CAD build for the part. Positions are in the model's coordinates, mm. Give positions to 0.01 mm unless a question says otherwise; leave off trailing zeros. Loops run counter-clockwise (first coordinate to the right, second up) from the corner with the lowest first, then second, coordinate; pieces in that order, holes last.
Item 1: Mould opens along Z. For faces 1 (the cylindrical face through (7.543, -2.415, 14.114)), 2 (the cylindrical face through (12.499, -2.348, 6.005)), 3 (the flat face through (50.377, -0.825, 15.654)) say: released by +Z, released by -Z, zero draft, split by the parting line, or undercut.
Item 2: Saw through at D-D on z = 15.5. Give the cut face in (x, y) (1 decimal), plus the area to 3 significant figures.
Item 3: Saw through at B-B on y = -3.75. Give the cut face in (x, z).
Item 4: Drop flat-ended pins along their axis: P1, Ø3.5, axis at x = 7.94, z = 11.11, coming from the -Y side; P2, Ø4, axis at x = 49, z = 11.5, coming from the +Y side. Give the stop position or say it passes through.
Item 5: Saw through at C-C on x = 47.5. Give the cut face in (y, z).
Item 6: Probe probe 1 along Z at (x, y) = (7, -0.9); probe 2 along Z at (x, y) = (8, -1.35); probe 3 along Z at (x, y) = (15, -1.8). List the from-to ranges inside material, lowest first.
Item 7: Saw through at A-A on z = 9.5. Give the cut face in (x, y), plus the area to 3 significant figures.
from build123d import *

# Parameters (mm, degrees)
F1_DEPTH = 4.7625
F2_R     = 3.027234
F3_DEPTH = 25.4
F5_DEPTH = 25.4


with BuildPart() as f1:
    # F0 (on Front) → F1 (new body)
    with BuildSketch(Plane.XZ):
        with BuildLine():
            Line((60.325, 19.05), (7.914832, 19.05))
            ThreePointArc((7.914832, 19.05), (2.318201, 16.731799), (0, 11.135168))
            Line((0, 11.135168), (0, 0))
            Line((0, 0), (9.520886, 0.27992))
            Line((9.520886, 0.27992), (10.734157, 3.685592))
            ThreePointArc((10.734157, 3.685592), (12.533664, 6.029149), (15.364371, 6.876249))
            Line((15.364371, 6.876249), (60.325, 12.7))
            Line((60.325, 12.7), (60.325, 19.05))
        make_face()
    extrude(amount=F1_DEPTH)

    # F2 (on face) → F3 (cut)
    with BuildSketch(Plane.XZ.offset(4.7625)):
        with Locations((7.937468, 11.1125)):
            Circle(F2_R)
    extrude(amount=-F3_DEPTH, mode=Mode.SUBTRACT)

    # F4 (on face) → F5 (cut)
    with BuildSketch(Plane.XY.offset(19.05)):
        Polygon((40.704425, 0), (60.325, -1.673274), (60.325, 0), align=None)
        Polygon((60.325, -4.7625), (60.325, -3.089226), (40.704425, -4.7625), align=None)
    extrude(amount=-F5_DEPTH, mode=Mode.SUBTRACT)


solid = f1.part
Results below:
1. face 1: undercut
1. face 2: released by -Z
1. face 3: zero draft
2. outline: (1.3, -4.8) - (40.7, -4.8) - (60.3, -3.1) - (60.3, -1.7) - (40.7, 0) - (1.3, 0) - close
2. area: 248 mm2
3. outline: (0, 0) - (9.52, 0.28) - (10.73, 3.69) arc R4.8 cw to (15.36, 6.88) - (52.58, 11.7) - (52.58, 19.05) - (7.91, 19.05) arc R7.91 ccw to (0, 11.14) - close; hole circle Ø6.05 at (7.94, 11.11)
4. P1: passes through
4. P2: stops at y = -0.54
5. outline: (-4.18, 11.04) - (-0.58, 11.04) - (-0.58, 19.05) - (-4.18, 19.05) - close
6. probe 1: z = 0.21 to 8.23, 13.99 to 19
6. probe 2: z = 0.24 to 8.09, 14.14 to 19.05
6. probe 3: z = 6.87 to 19.05
7. outline: (0, -4.76) - (5.38, -4.76) - (5.38, 0) - (0, 0) - close; (10.5, -4.76) - (35.62, -4.76) - (35.62, 0) - (10.5, 0) - close
7. area: 145 mm2
